Design review of the part shown in the three views and the two pictorial views. Dimensions are in mm from the part's minimum x, y and z. A direction names the side the tool comes from. Give positions to 0.01 mm unless a question says otherwise; leave off trailing zeros. Order: outer loops, then holes, each group sorted by start corner. A loop starts at its lowest first (then second) coordinate and runs counter-clockwise, first axis right, second up.
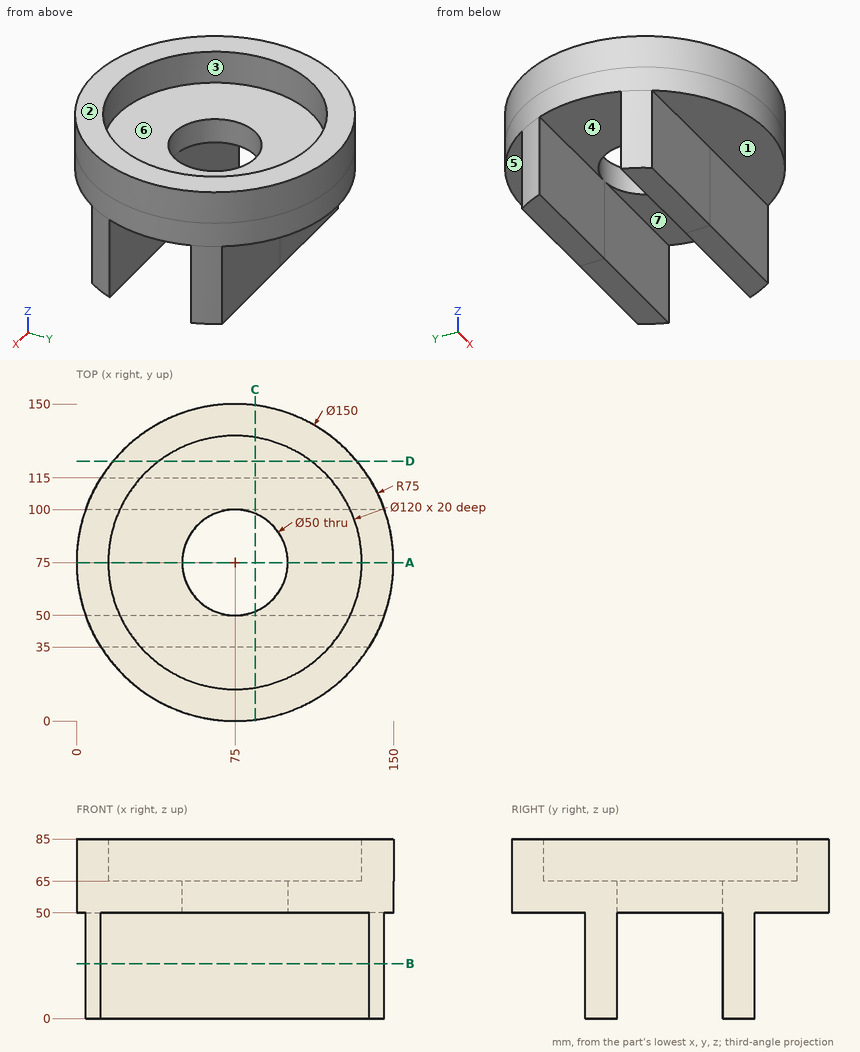
Item 1: Take a section at A-A (y = 75). Give the boundary of the cut face in (x, z).
Values found:
outline: (0, 50) - (50, 50) - (50, 65) - (15, 65) - (15, 85) - (0, 85) - close; (100, 50) - (150, 50) - (150, 85) - (135, 85) - (135, 65) - (100, 65) - close
Item 2: Take a section at D-D (y = 123). Give the boundary of the cut face in (x, z).
Values found:
outline: (17.37, 50) - (132.63, 50) - (132.63, 85) - (111, 85) - (111, 65) - (39, 65) - (39, 85) - (17.37, 85) - close
Item 3: Clearance check with flat-ended pins moving along their axes: pin 1 Ø6 at (x, z) = (133, 9) entering from +Y; pin 2 Ø10.5 at (x, y) = (103, 14.5) entering from -Z; pin 3 Ø1 at (x, y) = (104.5, 104.5) entering from +Z. State where each tip first meets the part, or that it passes through.
Values found:
pin 1: stops at y = 115
pin 2: stops at z = 50
pin 3: stops at z = 65
Item 4: For line 1 (Y direction, x = 129.5, z = 29); line 2 (Y direction, x = 75, z = 74.5); line 3 (Z direction, x = 74, y = 142), list the stretches that pass through material, from the lowest coordinate up.
Values found:
line 1: y = 35 to 50, 100 to 115
line 2: y = 0 to 15, 135 to 150
line 3: z = 50 to 85
Item 5: Draft analysis for pull direction X (two halves, no side actions). For the marked faces 6 and 7, state which applies: released by +X, released by -X, zero draft, split by the parting line, or undercut.
Values found:
face 6: undercut
face 7: zero draft
Item 6: For the marked faces 1, 2, 3, 4 and 5, list the 3-axis set-ups (+Z, -Z, +X, -X, +Y, -Y) from which the entire face can be reached by the end or side of a thin tool; tool diameter is ignored.
Values found:
face 1: -Z, +X, -X, -Y
face 2: +Z, +X, -X, +Y, -Y
face 3: +Z
face 4: -Z, +X, -X
face 5: -Z, +X, -X, +Y
Item 7: Take a section at C-C (x = 84.5). Give the boundary of the cut face in (y, z), and give its area (3 significant figures).
Values found:
outline: (0.6, 50) - (35, 50) - (35, 0) - (50, 0) - (50, 50) - (51.88, 50) - (51.88, 65) - (15.76, 65) - (15.76, 85) - (0.6, 85) - close; (98.12, 50) - (100, 50) - (100, 0) - (115, 0) - (115, 50) - (149.4, 50) - (149.4, 85) - (134.24, 85) - (134.24, 65) - (98.12, 65) - close
area: 3,640 mm2
Item 8: Take a section at B-B (z = 26). Give the boundary of the cut face in (x, y).
Values found:
outline: (4.29, 50) arc R75 ccw to (11.56, 35) - (138.44, 35) arc R75 ccw to (145.71, 50) - close; (4.29, 100) - (145.71, 100) arc R75 ccw to (138.44, 115) - (11.56, 115) arc R75 ccw to start
